Geometry: final body of the model. Coordinates: model frame, mm. Face numbers are marked on the shaded views. Round coordinates to 2 decimals unless told otherwise and drop trailing zeros. Loops run counter-clockwise (first coordinate to the right, second up) from the corner with the lowest first, then second, coordinate; pieces in that order, holes last. Notation, with made-up numbers: (-21.5, -36.75) - (4.5, -36.75) arc R24 ccw to (4.5, 0.25) - close; hole circle Ø7 at (-4.75, -4). An arc over 180 degrees is marked (long way). Use CSV: the item, a comma, the result in double quotes.
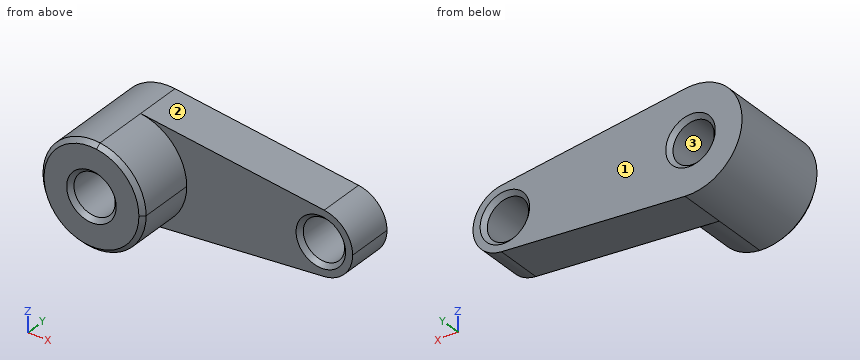
from build123d import *

# Parameters (mm, degrees)
F0_R     = 10
F2_DEPTH = 22
F3_DEPTH = 50
F4_SIZE  = 2


with BuildPart() as f2:
    # F0 (on Front) → F2 (new body)
    with BuildSketch(Plane.XZ):
        with BuildLine():
            ThreePointArc((2.656511, -24.858458), (18.593181, -16.71208), (25, 0))
            ThreePointArc((25, 0), (18.593181, 16.71208), (2.656511, 24.858458))
            ThreePointArc((2.656511, 24.858458), (-25, 0), (2.656511, -24.858458))
        make_face()
        Circle(F0_R, mode=Mode.SUBTRACT)
        with BuildLine():
            ThreePointArc((2.656511, 24.858458), (18.593181, 16.71208), (25, 0))
            ThreePointArc((25, 0), (18.593181, -16.71208), (2.656511, -24.858458))
            Line((2.656511, -24.858458), (91.640296, -15.349164))
            ThreePointArc((91.640296, -15.349164), (74.563439, 0), (91.640296, 15.349164))
            Line((91.640296, 15.349164), (2.656511, 24.858458))
        make_face()
        with BuildLine():
            ThreePointArc((105.436561, 0), (101.480591, 10.319081), (91.640296, 15.349164))
            ThreePointArc((91.640296, 15.349164), (74.563439, 0), (91.640296, -15.349164))
            ThreePointArc((91.640296, -15.349164), (101.480591, -10.319081), (105.436561, 0))
        make_face()
        with Locations((90, 0)):
            Circle(F0_R, mode=Mode.SUBTRACT)
    extrude(amount=F2_DEPTH)

    # F0 (on Front) → F3 (join)
    with BuildSketch(Plane.XZ):
        with BuildLine():
            ThreePointArc((2.656511, -24.858458), (18.593181, -16.71208), (25, 0))
            ThreePointArc((25, 0), (18.593181, 16.71208), (2.656511, 24.858458))
            ThreePointArc((2.656511, 24.858458), (-25, 0), (2.656511, -24.858458))
        make_face()
        Circle(F0_R, mode=Mode.SUBTRACT)
    extrude(amount=F3_DEPTH)

    # F4
    f4_edges = [f2.edges().sort_by_distance(p)[0] for p in [
        (80, -22, 0),
        (-10, -50, 0),
        (-2.656511, -50, 24.858458),
        (80, 0, 0),
        (-10, 0, 0),
    ]]
    chamfer(f4_edges, length=F4_SIZE)


solid = f2.part
Item 1: Pin query (flat end, axial travel): P1, Ø1.5, axis at x = 84.5, y = -17, coming from the +Z side; P2, Ø18, axis at x = 0, z = 0, coming from the +Y side; P3, Ø1.5, axis at y = -38.5, z = 7.5, coming from the +X side; P4, Ø3, axis at y = -25.5, z = -5.5, coming from the -X side. Return the tip coordinate at first contact, or that it passes through.
Final values:
P1,"stops at z = 16.19"
P2,"passes through"
P3,"stops at x = 24.07"
P4,"stops at x = -24.68"
Item 2: Section A-A on y = -11. Return the cut outline in (x, z).
Final values:
outline,"(2.66, -24.86) - (91.64, -15.35) arc R15.44 ccw to (105.44, 0) arc R15.44 ccw to (91.64, 15.35) - (2.66, 24.86) arc R25 ccw (long way) to start; hole circle Ø20 at (0, 0); hole circle Ø20 at (90, 0)"
Item 3: Section D-D on y = -43.5. Return the cut outline in (x, z), plus the area to 3 significant figures.
Final values:
outline,"circle Ø50 at (0, 0); hole circle Ø20 at (0, 0)"
area,"1,650 mm²"
Item 4: Material intervals for line 1 (Z direction, x = 0, y = -18); line 2 (Z direction, x = 90, y = -7); line 3 (Y direction, x = 72.5, z = 2), sorted ascending.
Final values:
line 1,"z = -25 to -10, 10 to 25"
line 2,"z = -15.52 to -10, 10 to 15.52"
line 3,"y = -22 to 0"
Item 5: Section B-B on x = 0. Return the cut outline in (y, z), plus the area to 3 significant figures.
Final values:
outline,"(-50, -23) - (-48, -25) - (0, -25) - (0, -12) - (-2, -10) - (-48, -10) - (-50, -12) - close; (-50, 12) - (-48, 10) - (-2, 10) - (0, 12) - (0, 25) - (-48, 25) - (-50, 23) - close"
area,"1,490 mm²"
Item 6: Mould query, pull axis Z, two halves, no side actions, for the marked faces 1, 2 and 3. Classes: released by +Z, released by -Z, zero draft, split by the parting line, or undercut.
Final values:
face 1,"zero draft"
face 2,"released by +Z"
face 3,"undercut"
Item 7: Section C-C on z = -5. Give the number of separate pieces and of enclosed holes in the cut face, plus the area to 3 significant figures.
Final values:
separate pieces,"3"
enclosed holes,"0"
area,"2,940 mm²"
